```python
from build123d import *

# Parameters (mm, degrees)
PAD003_DEPTH = 7
SKETCH002_R  = 1.5
PAD002_DEPTH = 15
SKETCH001_R  = 12
PAD001_DEPTH = 4
SKETCH004_R  = 1.5
PAD004_DEPTH = 14
PAD_DEPTH    = 14


with BuildPart() as obj1:
    # Sketch003 → Pad003 (new body)
    with BuildSketch(Plane.XZ.offset(-16)):
        Polygon((-13.4, 5.228719), (-11.8, 8), (-13.4, 10.771281), (-16.6, 10.771281), (-18.2, 8), (-16.6, 5.228719), align=None)
        Polygon((16.6, 5.228719), (18.2, 8), (16.6, 10.771281), (13.4, 10.771281), (11.8, 8), (13.4, 5.228719), align=None)
    extrude(amount=PAD003_DEPTH)


with BuildPart() as mount:
    # Sketch002 → Pad002 (new body)
    with BuildSketch(Plane.XZ):
        with Locations((-15, 8)):
            Circle(SKETCH002_R)
        with Locations((15, 8)):
            Circle(SKETCH002_R)
    extrude(amount=-PAD002_DEPTH)


with BuildPart() as obj2:
    # Sketch001 → Pad001 (new body)
    with BuildSketch(Plane.XY.offset(14)):
        Circle(SKETCH001_R)
    extrude(amount=-PAD001_DEPTH)


with BuildPart() as cutblock:
    # Sketch004 → Pad004 (new body)
    with BuildSketch(Plane.XY):
        with Locations((-5.974399, 5.689381)):
            Circle(SKETCH004_R)
        with Locations((5.974399, 5.689381)):
            Circle(SKETCH004_R)
        with Locations((-5.974399, -5.689381)):
            Circle(SKETCH004_R)
        with Locations((5.974399, -5.689381)):
            Circle(SKETCH004_R)
    extrude(amount=PAD004_DEPTH)

    # Fusion: union obj1, Mount, obj2
    add(obj1.part)
    add(mount.part)
    add(obj2.part)


with BuildPart() as cut:
    # Sketch → Pad (new body)
    with BuildSketch(Plane.XY):
        with BuildLine():
            ThreePointArc((5.2, 0), (0, 5.2), (-5.2, 0))
            Line((-20, 0), (-5.2, 0))
            ThreePointArc((20, 0), (0, 20), (-20, 0))
            Line((5.2, 0), (20, 0))
        make_face()
    extrude(amount=PAD_DEPTH)

    # Cut: cut CutBlock
    add(cutblock.part, mode=Mode.SUBTRACT)


solid = cut.part
```
Can you work these out from the model? Positions are in its coordinate system, mm. A direction names the side the tool comes from. Give positions to 0.01 mm unless a question says otherwise; leave off trailing zeros. Write each loop counter-clockwise with the first axis right and the second up, starting at its lowest first coordinate (ties: lowest second). Pieces come first, ordered by that corner, then holes. Notation, with made-up numbers: (27.25, -31.75) -> (76.25, -31.75) arc R21 cw to (76.25, -18.75) -> close; hole circle Ø8 at (50, -33.75). An arc over 180 degrees is marked (long way). One line per item, written item: value.
Q1. Which directions (+Z, -Z, +X, -X, +Y, -Y) give clear straight access to the entire face, cutting with the end or side of a thin tool? Please do faces 1 (the face through (-6.17, 7.177, 4.93)), 2 (the face through (15, 11, 10.771)).
Results found:
face 1: +Z, -Z
face 2: +Y
Q2. Imagine slicing it at A-A on z = 5.75. Please give me the cut outline in (x, y).
Results found:
outline: (-20, 0) -> (-5.2, 0) arc R5.2 cw to (5.2, 0) -> (20, 0) arc R20 ccw to (16.9, 10.69) -> (16.9, 9) -> (13.1, 9) -> (13.1, 15.11) arc R20 ccw to (-13.1, 15.11) -> (-13.1, 9) -> (-16.9, 9) -> (-16.9, 10.69) arc R20 ccw to start; hole circle Ø3 at (-5.97, 5.69); hole circle Ø3 at (5.97, 5.69)
Q3. For P1, Ø3, axis at x = 14, z = 7.5, coming from the +Y side; P2, Ø1, axis at y = 13.5, z = 7, coming from the +X side; P3, Ø6, axis at y = 9.5, z = 4.5, coming from the -X side, each with a flat end and sliding along its axis, tell me the tip position at first contact or that it passes through.
Results found:
P1: stops at y = 9
P2: stops at x = 12.67
P3: stops at x = -18.91
Q4. We'd pull the mould along Z, two halves only. Please class faces 3 (the face through (0, 10, 0)), 4 (the face through (12.59, 12.55, 6.63)), 5 (the face through (0, 12, 12)): +Z half, -Z half, draft (parallel to the pull), parting line (faces both ways), or undercut.
Results found:
face 3: -Z half
face 4: undercut
face 5: draft
Q5. Imagine slicing it at D-D on x = 0. Please give me the cut outline in (y, z).
Results found:
outline: (5.2, 0) -> (20, 0) -> (20, 14) -> (12, 14) -> (12, 10) -> (5.2, 10) -> close
Q6. Please list where these lines run through material, in increasing order: line 1 (X direction, y = 5.25, z = 4.5); line 2 (Z direction, x = -8, y = 1); line 3 (X direction, y = 2.75, z = 6). Write a range as [from, to].
Results found:
line 1: x = [-19.3, -7.41], [-4.54, 4.54], [7.41, 19.3]
line 2: z = [0, 10]
line 3: x = [-19.81, -4.41], [4.41, 19.81]
Q7. Imagine slicing it at C-C on x = 15. Please give me the cut outline in (y, z).
Results found:
outline: (0, 0) -> (13.23, 0) -> (13.23, 5.23) -> (9, 5.23) -> (9, 6.5) -> (0, 6.5) -> close; (0, 9.5) -> (9, 9.5) -> (9, 10.77) -> (13.23, 10.77) -> (13.23, 14) -> (0, 14) -> close
Q8. Imagine slicing it at B-B on y = 15.5. Please give me the cut outline in (x, z).
Results found:
outline: (-12.64, 0) -> (12.64, 0) -> (12.64, 6.55) -> (11.8, 8) -> (12.64, 9.45) -> (12.64, 14) -> (-12.64, 14) -> (-12.64, 9.45) -> (-11.8, 8) -> (-12.64, 6.55) -> close
